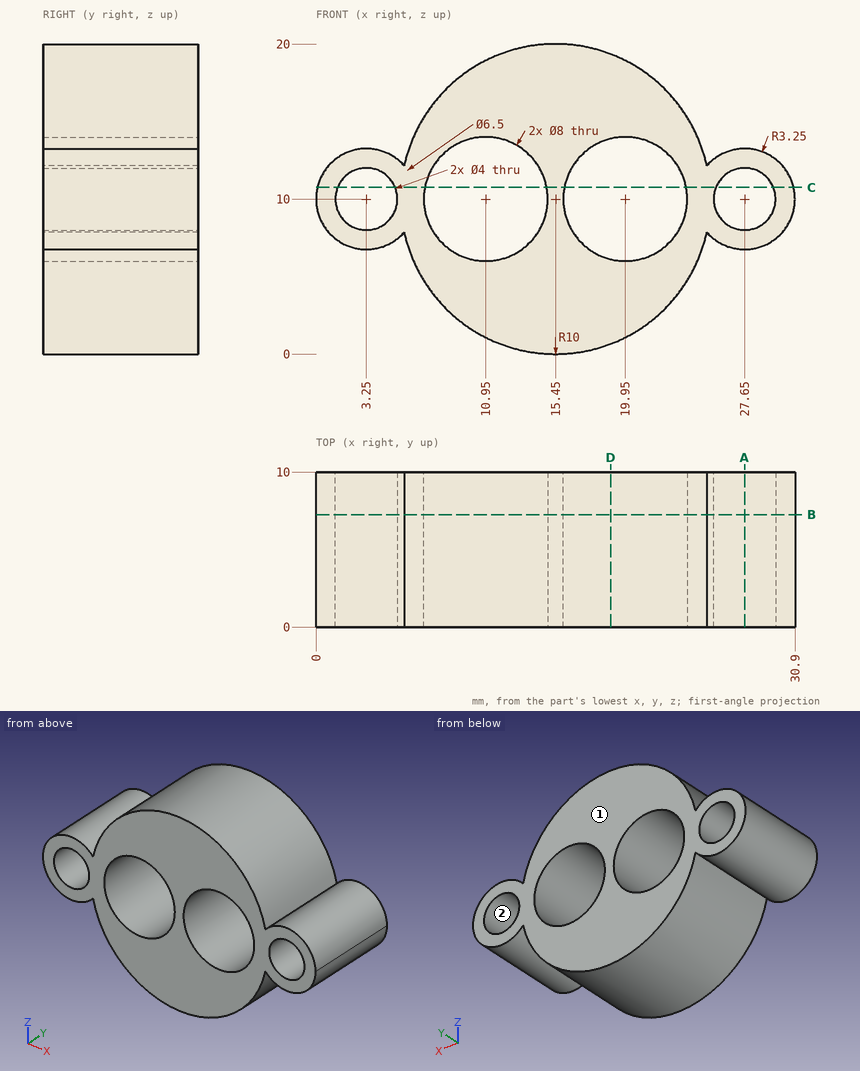
Check sheet for the drawn part. Datum: minimum x, y, z corner. Units: mm. Round coordinates to 2 decimals unless told otherwise and drop trailing zeros. Order: outer loops, then holes, each group sorted by start corner. A loop starts at its lowest first (then second) coordinate and runs counter-clockwise, first axis right, second up.
1) Scan lines: line 1 (X direction, y = 8.75, z = 11.5); line 2 (Z direction, x = 27.65, y = 4); line 3 (X direction, y = 2, z = 7). Record each from-to range of solid material in increasing order.
2) Section check A-A (x = 27.65). Record the boundary of the cut face in (y, z), and give its area (3 significant figures).
3) Section check D-D (x = 19). Record the boundary of the cut face in (y, z).
4) Mould release check, pull along Z, two halves, no side actions. Record for the marked faces 1 and 2: +Z half, -Z half, draft (parallel to the pull), parting line (faces both ways), or undercut.
5) Go/stop test with flat-tipped pins: pin 1 Ø1 at (x, y) = (24, 4) entering from +Z; pin 2 Ø3 at (y, z) = (4, 12) entering from -X; pin 3 Ø7 at (x, z) = (19.95, 10) entering from +Y; pin 4 Ø8 at (x, z) = (11.5, 12.5) entering from +Y. Record where each tip stops, or that it passes through.
6) Section check C-C (z = 10.75). Record the boundary of the cut face in (x, y).
7) Section check B-B (y = 7.25). Record the boundary of the cut face in (x, z).
Result:
1. line 1: x = 0.37 to 1.93, 4.57 to 7.24, 14.66 to 16.24, 23.66 to 26.33, 28.97 to 30.53
1. line 2: z = 6.75 to 8, 12 to 13.25
1. line 3: x = 2 to 4.5, 5.91 to 8.3, 13.6 to 17.3, 22.6 to 24.99, 26.4 to 28.9
2. outline: (0, 6.75) - (10, 6.75) - (10, 8) - (0, 8) - close; (0, 12) - (10, 12) - (10, 13.25) - (0, 13.25) - close
2. area: 25.0 mm2
3. outline: (0, 0.65) - (10, 0.65) - (10, 6.11) - (0, 6.11) - close; (0, 13.89) - (10, 13.89) - (10, 19.35) - (0, 19.35) - close
4. face 1: draft
4. face 2: undercut
5. pin 1: stops at z = 15.93
5. pin 2: stops at x = 0.04
5. pin 3: passes through
5. pin 4: stops at y = 10
6. outline: (0.09, 0) - (1.4, 0) - (1.4, 10) - (0.09, 10) - close; (5.1, 0) - (7.02, 0) - (7.02, 10) - (5.1, 10) - close; (14.88, 0) - (16.02, 0) - (16.02, 10) - (14.88, 10) - close; (23.88, 0) - (25.8, 0) - (25.8, 10) - (23.88, 10) - close; (29.5, 0) - (30.81, 0) - (30.81, 10) - (29.5, 10) - close
7. outline: (5.68, 7.85) arc R10 ccw to (25.22, 7.85) arc R3.25 ccw (long way) to (25.22, 12.15) arc R10 ccw to (5.68, 12.15) arc R3.25 ccw (long way) to start; hole circle Ø4 at (3.25, 10); hole circle Ø8 at (10.95, 10); hole circle Ø8 at (19.95, 10); hole circle Ø4 at (27.65, 10)
